```python
from build123d import *

# Parameters (mm, degrees)
SKETCH1_R           = 1.75
BOSS_EXTRUDE1_DEPTH = 6
CUT_EXTRUDE1_DEPTH  = 2.5
BOSS_EXTRUDE2_DEPTH = 6


with BuildPart() as part:
    # Sketch1 → Boss-Extrude1 (new body)
    with BuildSketch(Plane(origin=(0, 0, 0), x_dir=(1, 0, 0), z_dir=(0, 1, 0))):
        with BuildLine():
            Line((5, 0), (45, 0))
            ThreePointArc((45, 0), (48.535533906, 1.464466094), (50, 5))
            Line((50, 5), (50, 10))
            ThreePointArc((50, 10), (48.535533906, 13.535533906), (45, 15))
            Line((45, 15), (5, 15))
            ThreePointArc((5, 15), (1.464466094, 13.535533906), (0, 10))
            Line((0, 10), (0, 5))
            ThreePointArc((0, 5), (1.464466094, 1.464466094), (5, 0))
        make_face()
        with Locations((18.25, 7)):
            Circle(SKETCH1_R, mode=Mode.SUBTRACT)
        with Locations((31.75, 7)):
            Circle(SKETCH1_R, mode=Mode.SUBTRACT)
    boss_extrude1 = extrude(amount=BOSS_EXTRUDE1_DEPTH)

    # Sketch2 → Cut-Extrude1 (cut)
    with BuildSketch(Plane(origin=(0, 6, 0), x_dir=(1, 0, 0), z_dir=(0, 1, 0))):
        Polygon((19.83771324, 4.25), (21.425426481, 7), (19.83771324, 9.75), (16.66228676, 9.75), (15.074573519, 7), (16.66228676, 4.25), align=None)
        Polygon((33.33771324, 4.25), (34.925426481, 7), (33.33771324, 9.75), (30.16228676, 9.75), (28.574573519, 7), (30.16228676, 4.25), align=None)
    cut_extrude1 = extrude(amount=-CUT_EXTRUDE1_DEPTH, mode=Mode.SUBTRACT)

    # Mirror1: Boss-Extrude1, Cut-Extrude1 across plane
    add(boss_extrude1.mirror(Plane.XY))
    add(cut_extrude1.mirror(Plane.XY), mode=Mode.SUBTRACT)

    # Sketch3 → Boss-Extrude2 (add)
    with BuildSketch(Plane(origin=(0, 6, 0), x_dir=(1, 0, 0), z_dir=(0, 1, 0))):
        with BuildLine():
            Line((50, 5), (50, -5))
            ThreePointArc((50, -5), (48.535533906, -1.464466094), (45, 0))
            ThreePointArc((45, 0), (48.535533906, 1.464466094), (50, 5))
        make_face()
        with BuildLine():
            Line((0, 5), (0, -5))
            ThreePointArc((0, -5), (1.464466094, -1.464466094), (5, 0))
            ThreePointArc((5, 0), (1.464466094, 1.464466094), (0, 5))
        make_face()
    extrude(amount=-BOSS_EXTRUDE2_DEPTH)


solid = part.part
```
Source: CAD feature listing. Evaluate the final solid. Frame: model axes, mm. A direction names the side the tool comes from. Coordinates: 2 decimals unless noted, no trailing zeros. Order: outer loops, then holes, each group sorted by start corner. A loop starts at its lowest first (then second) coordinate and runs counter-clockwise, first axis right, second up. Notation, with made-up numbers: (72.25, -22.75) - (101.25, -22.75) arc R19 ccw to (101.25, 4.25) - close; hole circle Ø10 at (-19, -10). An arc over 180 degrees is marked (long way). One line per item, written item: value.
1) Cut plane A-A on x = 31.75. Output: boundary loops of the cut face in (y, z), plus the area to 3 significant figures.
Computed values:
outline: (0, -15) - (6, -15) - (6, -9.75) - (3.5, -9.75) - (3.5, -8.75) - (0, -8.75) - close; (0, -5.25) - (3.5, -5.25) - (3.5, -4.25) - (6, -4.25) - (6, 4.25) - (3.5, 4.25) - (3.5, 5.25) - (0, 5.25) - close; (0, 8.75) - (3.5, 8.75) - (3.5, 9.75) - (6, 9.75) - (6, 15) - (0, 15) - close
area: 128 mm^2
2) Reachability of faces 1 (the face through (49, 3, -13)), 2 (the face through (18, 5, -9.75)) from +Z, -Z, +X, -X, +Y, -Y: full face, straight path, thin tool, end or side. Return the list, or none.
Computed values:
face 1: -Z, +X, +Y, -Y
face 2: +Y
3) Contact query for flat-ended pins moving along their axis: pin 1 (3 mm diameter, centred on x = 32.5, z = -6.5, fed in from +Y); pin 2 (3 mm diameter, centred on x = 31.75, z = 7, fed in from +Y); pin 3 (6 mm diameter, centred on x = 19.5, z = -7.5, fed in from +Y). Output: stop coordinate, or through.
Computed values:
pin 1: stops at y = 3.5
pin 2: passes through
pin 3: stops at y = 6
4) Cut plane D-D on y = 5.35. State how many separate pieces and enclosed holes the cut face has, plus the area to 3 significant figures.
Computed values:
separate pieces: 1
enclosed holes: 4
area: 1,370 mm^2
5) Cut plane C-C on z = 9.25. Output: boundary loops of the cut face in (x, y), plus the area to 3 significant figures.
Computed values:
outline: (0, 0) - (50, 0) - (50, 6) - (33.63, 6) - (33.63, 3.5) - (29.87, 3.5) - (29.87, 6) - (20.13, 6) - (20.13, 3.5) - (16.37, 3.5) - (16.37, 6) - (0, 6) - close
area: 281 mm^2
6) Cut plane B-B on y = 1.15. Output: boundary loops of the cut face in (x, z), plus the area to 3 significant figures.
Computed values:
outline: (0, -10) arc R5 ccw to (5, -15) - (45, -15) arc R5 ccw to (50, -10) - (50, 10) arc R5 ccw to (45, 15) - (5, 15) arc R5 ccw to (0, 10) - close; hole circle Ø3.5 at (18.25, -7); hole circle Ø3.5 at (18.25, 7); hole circle Ø3.5 at (31.75, -7); hole circle Ø3.5 at (31.75, 7)
area: 1,440 mm^2
7) Ray query, line 1 (Z direction, x = 18.25, y = 0.9); line 2 (X direction, y = 0.9, z = -7); line 3 (Y direction, x = 29, z = -7.25). Return the intervals inside material, ascending. Write a range as [from, to].
Computed values:
line 1: z = [-15, -8.75], [-5.25, 5.25], [8.75, 15]
line 2: x = [0, 16.5], [20, 30], [33.5, 50]
line 3: y = [0, 3.5]
8) Mould query, pull axis X, two halves, no side actions, for faces 3 (the face through (29.38, 4.768, -8.394)), 4 (the face through (2, 3, -14)), 5 (the face through (49, 3, 13)). Classes: released by +X, released by -X, zero draft, split by the parting line, or undercut.
Computed values:
face 3: undercut
face 4: released by -X
face 5: released by +X
